Verification items for the finished model (mm, model axes). A direction names the side the tool comes from. Give positions to 0.01 mm unless a question says otherwise; leave off trailing zeros. Order: outer loops, then holes, each group sorted by start corner. A loop starts at its lowest first (then second) coordinate and runs counter-clockwise, first axis right, second up. Notation, with made-up numbers: (70.5, 50) - (83.5, 50) arc R29 cw to (83.5, 89) - close; hole circle Ø3 at (13, 51.5). An arc over 180 degrees is marked (long way). Answer as a JSON object with one key per item and string values. Group by question number.
(1) Section check B-B (z = 8). Record the boundary of the cut face in (x, y), then the cut area to 3 significant figures.
(2) Access from +Z, -Z, +X, -X, +Y, -Y to the whole of each face (thin tool, end or side, straight path). Record for faces 1 (the face through (13.07, 0.99, -7.5)), 2 (the face through (-0.4, 2, -9.2)), 3 (the face through (0, 1, 20)).
(3) Depth check by flat-ended pin: pin 1 Ø1.5 at (x, y) = (8.5, 3.5) entering from -Z; pin 2 Ø4 at (x, z) = (18.5, 8) entering from +Y. Enter the tip coordinate at first touch or a pass-through.
(4) Section check D-D (z = -15). Record the boundary of the cut face in (x, y), then the cut area to 3 significant figures.
(5) Section check C-C (x = 1.5). Record the boundary of the cut face in (y, z), then the cut area to 3 significant figures.
(6) Thickness scan on line 1 (X direction, y = 4.6, z = -15); line 2 (X direction, y = 3.55, z = -5.5) (3 decimals); line 3 (Z direction, x = 3, y = 0.85). Record the ranges inside material, lowest first.
(7) Mould release check, pull along Z, two halves, no side actions. Record for faces 4 (the face through (0, 1, -9)), 5 (the face through (-6.9, 6, -15)), 6 (the face through (22.863, 3.042, -5.679)), 7 (the face through (-15.87, 1.01, -19.61)): +Z half, -Z half, draft (parallel to the pull), parting line (faces both ways), or undercut.
(8) Section check A-A (y = 4.4). Count the separate pieces of the cut face and the enclosed holes in it, then the cut area to 3 significant figures.
```python
from build123d import *

# Parameters (mm, degrees)
SKETCH1_W           = 52
SKETCH1_H           = 40
BOSS_EXTRUDE1_DEPTH = 2
SKETCH2_R           = 0.9
SKETCH2_R_2         = 1.375
CUT_EXTRUDE1_DEPTH  = 33.86335345
BOSS_EXTRUDE2_START = 4
SKETCH3_R           = 3.5
SKETCH3_R_2         = 1.375
SKETCH3_R_3         = 2.5
SKETCH3_R_4         = 0.9
BOSS_EXTRUDE2_DEPTH = 4
SKETCH4_W           = 29
SKETCH4_H           = 25.5
CUT_EXTRUDE2_DEPTH  = 34.045423284
CHAMFER1_SIZE       = 10
FILLET1_R           = 5


with BuildPart() as part:
    # Sketch1 → Boss-Extrude1 (new body)
    with BuildSketch(Plane(origin=(0, 0, 0), x_dir=(1, 0, 0), z_dir=(0, 1, 0))):
        Rectangle(SKETCH1_W, SKETCH1_H)
    extrude(amount=BOSS_EXTRUDE1_DEPTH)

    # Sketch2 → Cut-Extrude1 (cut, through all)
    with BuildSketch(Plane(origin=(0, 2, 0), x_dir=(1, 0, 0), z_dir=(0, 1, 0))):
        with Locations(Location((8, 15, 0), (0, 0, 270))):
            Circle(SKETCH2_R)
        with Locations(Location((-8, 15, 0), (0, 0, 270))):
            Circle(SKETCH2_R)
        with Locations(Location((-21.5, 5.5, 0), (0, 0, 270))):
            Circle(SKETCH2_R_2)
        with Locations(Location((-21.5, -15, 0), (0, 0, 270))):
            Circle(SKETCH2_R_2)
        with Locations(Location((21.5, -15, 0), (0, 0, 270))):
            Circle(SKETCH2_R_2)
        with Locations(Location((21.5, 5.5, 0), (0, 0, 270))):
            Circle(SKETCH2_R_2)
    extrude(amount=-CUT_EXTRUDE1_DEPTH, mode=Mode.SUBTRACT)

    # Sketch3 → Boss-Extrude2 (add)
    # profile 1 of 6: a face of its own
    with BuildSketch(Plane(origin=(0, 2, 0), x_dir=(1, 0, 0), z_dir=(0, 1, 0)).offset(BOSS_EXTRUDE2_START)):
        with Locations(Location((-21.5, 5.5, 0), (0, 0, 90))):
            Circle(SKETCH3_R)
        with Locations(Location((-21.5, 5.5, 0), (0, 0, 270))):
            Circle(SKETCH3_R_2, mode=Mode.SUBTRACT)
    # profile 2 of 6: a face of its own
    with BuildSketch(Plane(origin=(0, 2, 0), x_dir=(1, 0, 0), z_dir=(0, 1, 0)).offset(BOSS_EXTRUDE2_START)):
        with Locations(Location((-21.5, -15, 0), (0, 0, 90))):
            Circle(SKETCH3_R)
        with Locations(Location((-21.5, -15, 0), (0, 0, 270))):
            Circle(SKETCH3_R_2, mode=Mode.SUBTRACT)
    # profile 3 of 6: a face of its own
    with BuildSketch(Plane(origin=(0, 2, 0), x_dir=(1, 0, 0), z_dir=(0, 1, 0)).offset(BOSS_EXTRUDE2_START)):
        with Locations(Location((21.5, -15, 0), (0, 0, 90))):
            Circle(SKETCH3_R)
        with Locations(Location((21.5, -15, 0), (0, 0, 270))):
            Circle(SKETCH3_R_2, mode=Mode.SUBTRACT)
    # profile 4 of 6: a face of its own
    with BuildSketch(Plane(origin=(0, 2, 0), x_dir=(1, 0, 0), z_dir=(0, 1, 0)).offset(BOSS_EXTRUDE2_START)):
        with Locations(Location((21.5, 5.5, 0), (0, 0, 90))):
            Circle(SKETCH3_R)
        with Locations(Location((21.5, 5.5, 0), (0, 0, 270))):
            Circle(SKETCH3_R_2, mode=Mode.SUBTRACT)
    # profile 5 of 6: a face of its own
    with BuildSketch(Plane(origin=(0, 2, 0), x_dir=(1, 0, 0), z_dir=(0, 1, 0)).offset(BOSS_EXTRUDE2_START)):
        with Locations(Location((8, 15, 0), (0, 0, 90))):
            Circle(SKETCH3_R_3)
        with Locations(Location((8, 15, 0), (0, 0, 270))):
            Circle(SKETCH3_R_4, mode=Mode.SUBTRACT)
    # profile 6 of 6: a face of its own
    with BuildSketch(Plane(origin=(0, 2, 0), x_dir=(1, 0, 0), z_dir=(0, 1, 0)).offset(BOSS_EXTRUDE2_START)):
        with Locations(Location((-8, 15, 0), (0, 0, 90))):
            Circle(SKETCH3_R_3)
        with Locations(Location((-8, 15, 0), (0, 0, 270))):
            Circle(SKETCH3_R_4, mode=Mode.SUBTRACT)
    extrude(amount=-BOSS_EXTRUDE2_DEPTH)

    # Sketch4 → Cut-Extrude2 (cut, through all)
    with BuildSketch(Plane(origin=(0, 2, 0), x_dir=(1, 0, 0), z_dir=(0, 1, 0))):
        with Locations((0, -3.75)):
            Rectangle(SKETCH4_W, SKETCH4_H)
    extrude(amount=-CUT_EXTRUDE2_DEPTH, mode=Mode.SUBTRACT)

    # Chamfer1
    chamfer1_edges = [part.edges().sort_by_distance(p)[0] for p in [
        (-26, 1, -20),
        (26, 1, -20),
    ]]
    chamfer(chamfer1_edges, length=CHAMFER1_SIZE)

    # Fillet1
    fillet1_edges = [part.edges().sort_by_distance(p)[0] for p in [
        (26, 1, 20),
        (-26, 1, 20),
        (14.5, 1, -9),
        (14.5, 1, 16.5),
        (-14.5, 1, 16.5),
        (-14.5, 1, -9),
        (-16, 1, -20),
        (16, 1, -20),
        (26, 1, -10),
        (-26, 1, -10),
    ]]
    fillet(fillet1_edges, radius=FILLET1_R)


solid = part.part
```
Solutions:
{
 "1": {"outline": "(-26, 0) - (-14.5, 0) - (-14.5, 2) - (-26, 2) - close; (14.5, 0) - (26, 0) - (26, 2) - (14.5, 2) - close", "area": "46.0 mm2"},
 "2": {"face 1": "+Y, -Y", "face 2": "+Y", "face 3": "+Z, +X, -X, +Y, -Y"},
 "3": {"pin 1": "stops at z = -17.5", "pin 2": "stops at y = 2"},
 "4": {"outline": "(-21, 0) - (-8.9, 0) - (-8.9, 6) - (-10.5, 6) - (-10.5, 2) - (-21, 2) - close; (-7.1, 0) - (7.1, 0) - (7.1, 6) - (5.5, 6) - (5.5, 2) - (-5.5, 2) - (-5.5, 6) - (-7.1, 6) - close; (8.9, 0) - (21, 0) - (21, 2) - (10.5, 2) - (10.5, 6) - (8.9, 6) - close", "area": "102 mm2"},
 "5": {"outline": "(0, -20) - (2, -20) - (2, -9) - (0, -9) - close; (0, 16.5) - (2, 16.5) - (2, 20) - (0, 20) - close", "area": "29.0 mm2"},
 "6": {"line 1": "x = -10.5 to -8.9, -7.1 to -5.5, 5.5 to 7.1, 8.9 to 10.5", "line 2": "x = -25 to -22.875, -20.125 to -18, 18 to 20.125, 22.875 to 25", "line 3": "z = -20 to -9, 16.5 to 20"},
 "7": {"face 4": "undercut", "face 5": "draft", "face 6": "undercut", "face 7": "-Z half"},
 "8": {"separate pieces": "6", "enclosed holes": "6", "area": "164 mm2"}
}
